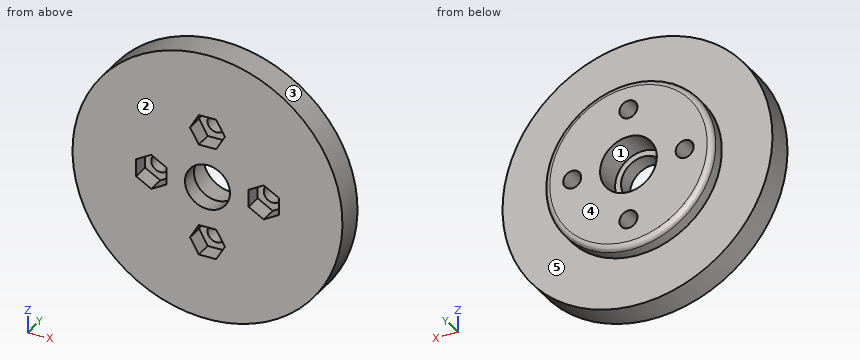
from build123d import *

# Parameters (mm, degrees)
SKETCH1_R           = 24
SKETCH1_R_2         = 4
BOSS_EXTRUDE1_DEPTH = 5
SKETCH2_R           = 15
BOSS_EXTRUDE2_DEPTH = 3
SKETCH4_R           = 5.05
CUT_EXTRUDE2_DEPTH  = 5
FILLET1_R           = 1
SKETCH5_R           = 1.6
CUT_EXTRUDE3_DEPTH  = 35.871191548
CUT_EXTRUDE15_DEPTH = 3


with BuildPart() as part:
    # Sketch1 → Boss-Extrude1 (new body)
    with BuildSketch(Plane(origin=(0, 0, 0), x_dir=(1, 0, 0), z_dir=(0, 1, 0))):
        with Locations(Location((0, 0, 0), (0, 0, 270))):
            Circle(SKETCH1_R)
        with Locations(Location((0, 0, 0), (0, 0, 270))):
            Circle(SKETCH1_R_2, mode=Mode.SUBTRACT)
    extrude(amount=BOSS_EXTRUDE1_DEPTH)

    # Sketch2 → Boss-Extrude2 (add)
    with BuildSketch(Plane(origin=(0, 5, 0), x_dir=(1, 0, 0), z_dir=(0, 1, 0))):
        with Locations(Location((0, 0, 0), (0, 0, 270))):
            Circle(SKETCH2_R)
    extrude(amount=BOSS_EXTRUDE2_DEPTH)

    # Sketch4 → Cut-Extrude2 (cut)
    with BuildSketch(Plane(origin=(0, 8, 0), x_dir=(1, 0, 0), z_dir=(0, 1, 0))):
        with Locations(Location((0, 0, 0), (0, 0, 270))):
            Circle(SKETCH4_R)
    extrude(amount=-CUT_EXTRUDE2_DEPTH, mode=Mode.SUBTRACT)

    # Fillet1
    fillet1_edges = [part.edges().sort_by_distance(p)[0] for p in [
        (0, 8, -15),
    ]]
    fillet(fillet1_edges, radius=FILLET1_R)

    # Sketch5 → Cut-Extrude3 (cut, through all)
    with BuildSketch(Plane(origin=(0, 8, 0), x_dir=(1, 0, 0), z_dir=(0, 1, 0))):
        with Locations(Location((0, 10, 0), (0, 0, 270))):
            Circle(SKETCH5_R)
        with Locations(Location((-10, 0, 0), (0, 0, 270))):
            Circle(SKETCH5_R)
        with Locations(Location((0, -10, 0), (0, 0, 270))):
            Circle(SKETCH5_R)
        with Locations(Location((10, 0, 0), (0, 0, 270))):
            Circle(SKETCH5_R)
    extrude(amount=-CUT_EXTRUDE3_DEPTH, mode=Mode.SUBTRACT)

    # Sketch10 → Cut-Extrude15 (cut)
    with BuildSketch(Plane.XZ):
        Polygon((10, -3.1), (12.684678752, -1.55), (12.684678752, 1.55), (10, 3.1), (7.315321248, 1.55), (7.315321248, -1.55), align=None)
        Polygon((3.1, 10), (1.55, 12.684678752), (-1.55, 12.684678752), (-3.1, 10), (-1.55, 7.315321248), (1.55, 7.315321248), align=None)
        Polygon((-3.1, -10), (-1.55, -12.684678752), (1.55, -12.684678752), (3.1, -10), (1.55, -7.315321248), (-1.55, -7.315321248), align=None)
        Polygon((-10, 3.1), (-12.684678752, 1.55), (-12.684678752, -1.55), (-10, -3.1), (-7.315321248, -1.55), (-7.315321248, 1.55), align=None)
    extrude(amount=-CUT_EXTRUDE15_DEPTH, mode=Mode.SUBTRACT)


solid = part.part
Source: CAD feature listing. Evaluate the final solid. Frame: model axes, mm. Face numbers are marked on the shaded views. A direction names the side the tool comes from. Give positions to 0.01 mm unless a question says otherwise; leave off trailing zeros. Write each loop counter-clockwise with the first axis right and the second up, starting at its lowest first coordinate (ties: lowest second). Pieces come first, ordered by that corner, then holes. Notation, with made-up numbers: (-7.5, 86) - (0.5, 86) arc R20 ccw to (0.5, 95) - close; hole circle Ø4 at (28.25, 81.5). An arc over 180 degrees is marked (long way). Write item = value, one per line. Start each with the question number.
Q1. Pin query (flat end, axial travel): pin 1 Ø3 at (x, z) = (0, -10) entering from -Y; pin 2 Ø1.5 at (y, z) = (1, 0.5) entering from -X; pin 3 Ø1.5 at (x, y) = (3, 5.5) entering from +Z; pin 4 Ø2 at (x, y) = (-7.5, 7) entering from +Z. Return the tip coordinate at first contact, or that it passes through.
Q2. Reachability of the marked faces 4 and 5 from +Z, -Z, +X, -X, +Y, -Y: full face, straight path, thin tool, end or side. Return the list, or none.
Q3. Cut plane D-D, the plane z = -18. Return loops of the section in (x, y).
Q4. Cut plane C-C, the plane y = 1.5. Return loops of the section in (x, z), then the cut area to 3 significant figures.
Q5. Material intervals for probe 1 along X at (y, z) = (0.75, 0); probe 2 along X at (y, z) = (4.95, 0); probe 3 along Y at (x, z) = (0.5, -19.5), sorted ascending.
Q6. Cut plane A-A, the plane x = 0. Give the number of separate pieces and of enclosed holes in the cut face, then the cut area to 3 significant figures.
Q7. Draft query along X for the marked faces 1, 2 and 3. Return one class per face: +X half, -X half, draft (parallel to the pull), parting line (faces both ways), or undercut.
Computed values:
q1.pin_1 = through
q1.pin_2 = -24
q1.pin_3 = 23.88
q1.pin_4 = 13.52
q2.face_4 = +Z, -Z, +X, -X, +Y
q2.face_5 = +Y
q3.outline = (-15.87, 0) - (15.87, 0) - (15.87, 5) - (-15.87, 5) - close
q4.outline = circle Ø48 at (0, 0); hole (-12.68, -1.55) - (-10, -3.1) - (-7.32, -1.55) - (-7.32, 1.55) - (-10, 3.1) - (-12.68, 1.55) - close; hole circle Ø8 at (0, 0); hole (-3.1, -10) - (-1.55, -12.68) - (1.55, -12.68) - (3.1, -10) - (1.55, -7.32) - (-1.55, -7.32) - close; hole (-3.1, 10) - (-1.55, 7.32) - (1.55, 7.32) - (3.1, 10) - (1.55, 12.68) - (-1.55, 12.68) - close; hole (7.32, -1.55) - (10, -3.1) - (12.68, -1.55) - (12.68, 1.55) - (10, 3.1) - (7.32, 1.55) - close
q4.area = 1,660 mm²
q5.probe_1 = -24 to -12.68, -7.32 to -4, 4 to 7.32, 12.68 to 24
q5.probe_2 = -24 to -11.6, -8.4 to -5.05, 5.05 to 8.4, 11.6 to 24
q5.probe_3 = 0 to 5
q6.separate_pieces = 4
q6.enclosed_holes = 0
q6.area = 191 mm²
q7.face_1 = undercut
q7.face_2 = draft
q7.face_3 = parting line
